For this review, take the finished solid that the model builds, in its own axes (mm). A direction names the side the tool comes from. Coordinates: 2 decimals unless noted, no trailing zeros. Order: outer loops, then holes, each group sorted by start corner. A loop starts at its lowest first (then second) coordinate and runs counter-clockwise, first axis right, second up.
from build123d import *

# Parameters (mm, degrees)
F0_R     = 2
F1_DEPTH = 5
F2_DEPTH = 30
F3_START = 25
F3_DEPTH = 5


with BuildPart() as f1:
    # F0 (on Top) → F1 (new body)
    with BuildSketch(Plane.XY):
        Circle(F0_R)
    extrude(amount=F1_DEPTH)

    # F0 (on Top) → F2 (join)
    with BuildSketch(Plane.XY):
        Polygon((0, 18), (-15.5884572681, 9), (-15.5884572681, -9), (0, -18), (15.5884572681, -9), (15.5884572681, 9), (10.1517191776, 12.1389022001), (10.1517191776, 8.1389022001), (1.4914651398, 13.1389022001), (4.9555667549, 15.1389022001), align=None)
        Circle(F0_R, mode=Mode.SUBTRACT)
    extrude(amount=F2_DEPTH)

    # F0 (on Top) → F3 (join)
    with BuildSketch(Plane.XY.offset(F3_START)):
        Polygon((10.1517191776, 12.1389022001), (4.9555667549, 15.1389022001), (1.4914651398, 13.1389022001), (10.1517191776, 8.1389022001), align=None)
    extrude(amount=F3_DEPTH)


solid = f1.part
1. Take a section at C-C, the plane y = 0. Give the boundary of the cut face in (x, z), plus the area to 3 significant figures.
Answer below:
outline: (-15.59, 0) - (15.59, 0) - (15.59, 30) - (2, 30) - (2, 5) - (-2, 5) - (-2, 30) - (-15.59, 30) - close
area: 835 mm2
2. Take a section at D-D, the plane x = 6. Give the boundary of the cut face in (y, z).
Answer below:
outline: (-14.54, 0) - (10.54, 0) - (10.54, 25) - (14.54, 25) - (14.54, 30) - (-14.54, 30) - close
3. Take a section at A-A, the plane z = 19.5. Give the boundary of the cut face in (x, y), plus the area to 3 significant figures.
Answer below:
outline: (-15.59, -9) - (0, -18) - (15.59, -9) - (15.59, 9) - (10.15, 12.14) - (10.15, 8.14) - (1.49, 13.14) - (4.96, 15.14) - (0, 18) - (-15.59, 9) - close; hole circle Ø4 at (0, 0)
area: 801 mm2
4. Take a section at B-B, the plane z = 2. Give the boundary of the cut face in (x, y), plus the area to 3 significant figures.
Answer below:
outline: (-15.59, -9) - (0, -18) - (15.59, -9) - (15.59, 9) - (10.15, 12.14) - (10.15, 8.14) - (1.49, 13.14) - (4.96, 15.14) - (0, 18) - (-15.59, 9) - close
area: 814 mm2
5. Machinability: for faces 1 (the face through (5.882, 10.604, 12.325)), 2 (the face through (15.588, 0, 15)), 3 (the face through (3.199, 14.125, 12.325)), 4 (the face through (0, -2, 17)), which of the approach directions +Z, -Z, +X, -X, +Y, -Y give a long, thin tool a straight path to every point of the face, cutting with its end or side? Answer none if there is none.
Answer below:
face 1: -Z
face 2: +Z, -Z, +X, +Y, -Y
face 3: -Z, +X
face 4: +Z
6. Clearance check with flat-ended pins moving along their axes: pin 1 Ø1.2 at (x, y) = (0, 0.5) entering from +Z; pin 2 Ø1.2 at (y, z) = (10.5, 8) entering from -X; pin 3 Ø3 at (x, z) = (-3.5, 4.5) entering from -Y. State where each tip first meets the part, or that it passes through.
Answer below:
pin 1: stops at z = 5
pin 2: stops at x = -14.03
pin 3: stops at y = -16.85
7. The part is to be moulded in two halves that separate along Y. For faces 5 (the face through (10.152, 10, 12)), 6 (the face through (7.69, -13.56, 14.79)), 7 (the face through (0, 0, 5)), say which applies: +Y half, -Y half, draft (parallel to the pull), parting line (faces both ways), or undercut.
Answer below:
face 5: draft
face 6: -Y half
face 7: undercut
8. To check wall thickness, follow L1, parallel to Y at x = 0, z = 20.25; L2, parallel to Y at x = 2.5, z = 5.5; L3, parallel to Y at x = -8.5, z = 28.25. State the ranges of each line that lie inside material, in increasing order.
Answer below:
L1: y = -18 to -2, 2 to 18
L2: y = -16.56 to 12.56, 13.72 to 16.56
L3: y = -13.09 to 13.09
